Source: CAD feature listing. Evaluate the final solid. Frame: model axes, mm. A direction names the side the tool comes from. Coordinates: 2 decimals unless noted, no trailing zeros. Order: outer loops, then holes, each group sorted by start corner. A loop starts at its lowest first (then second) coordinate and runs counter-clockwise, first axis right, second up. Notation, with made-up numbers: (-37.75, 36.5) -> (-28.75, 36.5) arc R27 ccw to (-28.75, 75.5) -> close; hole circle Ø8 at (-12.75, -26). An arc over 180 degrees is marked (long way). Put each result on its own line as item: value.
from build123d import *

# Parameters (mm, degrees)
SKETCH_1_W                   = 38
SKETCH_1_H                   = 6.45
EXTRUDE_1_DEPTH              = 35
SKETCH_2_W                   = 10
SKETCH_2_H                   = 35
EXTRUDE_2_DEPTH              = 15
HOLE_WIZARD_M4_1_D           = 4.5
HOLE_WIZARD_M4_1_CBORE_D     = 8
HOLE_WIZARD_M4_1_CBORE_DEPTH = 4
PATTERN_LINEAR_1_COUNT       = 2
PATTERN_LINEAR_1_PITCH       = 11
SKETCH_5_R                   = 2
CUT_EXTRUDE_1_DEPTH          = 54.795910625
SKETCH_6_R                   = 2
CUT_EXTRUDE_2_DEPTH          = 56.938381278
PATTERN_LINEAR_2_COUNT       = 2
PATTERN_LINEAR_2_PITCH       = 28
PATTERN_LINEAR_2_COUNT_DIR2  = 2
PATTERN_LINEAR_2_PITCH_DIR2  = 25
CHAMFER_1_SIZE               = 0.5


with BuildPart() as part:
    # 草图1 → 凸台-拉伸1 (new body)
    with BuildSketch(Plane.XY):
        with Locations((19, 3.225)):
            Rectangle(SKETCH_1_W, SKETCH_1_H)
    extrude(amount=EXTRUDE_1_DEPTH)

    # 草图2 → 凸台-拉伸2 (add)
    with BuildSketch(Plane(origin=(0, 6.45, 0), x_dir=(1, 0, 0), z_dir=(0, 1, 0))):
        with Locations((5, -17.5)):
            Rectangle(SKETCH_2_W, SKETCH_2_H)
        with Locations((33, -17.5)):
            Rectangle(SKETCH_2_W, SKETCH_2_H)
    extrude(amount=EXTRUDE_2_DEPTH)

    # Hole Wizard M4 _1 (through all)
    with Locations(Plane(origin=(0, 21.45, 0), x_dir=(-1, 0, 0), z_dir=(0, 1, 0))):
        with Locations((-5, 23)):
            hole_wizard_m4_1 = CounterBoreHole(HOLE_WIZARD_M4_1_D / 2, HOLE_WIZARD_M4_1_CBORE_D / 2, HOLE_WIZARD_M4_1_CBORE_DEPTH)

    # 阵列(线性)1: Hole Wizard M4 _1 ×2
    with Locations(*[(0, 0, -i * PATTERN_LINEAR_1_PITCH) for i in range(1, PATTERN_LINEAR_1_COUNT)]):
        add(hole_wizard_m4_1, mode=Mode.SUBTRACT)

    # 草图5 → 切除-拉伸1 (cut, through all)
    with BuildSketch(Plane(origin=(0, 6.45, 0), x_dir=(1, 0, 0), z_dir=(0, 1, 0))):
        with Locations(Location((19, -27.5, 0), (0, 0, 180))):
            Circle(SKETCH_5_R)
        with Locations(Location((19, -7.5, 0), (0, 0, 180))):
            Circle(SKETCH_5_R)
    extrude(amount=-CUT_EXTRUDE_1_DEPTH, mode=Mode.SUBTRACT)

    # 草图6 → 切除-拉伸2 (cut, through all)
    with BuildSketch(Plane(origin=(0, 21.45, 0), x_dir=(1, 0, 0), z_dir=(0, 1, 0))):
        with Locations(Location((33, -23, 0), (0, 0, 270))):
            Circle(SKETCH_6_R)
        with Locations(Location((33, -12, 0), (0, 0, 270))):
            Circle(SKETCH_6_R)
    extrude(amount=-CUT_EXTRUDE_2_DEPTH, mode=Mode.SUBTRACT)

    # 草图7 → Hole Wizard M4 _1 2 (revolve, cut)
    with BuildSketch(Plane(origin=(5, 21.45, 30), x_dir=(0, 0, 1), z_dir=(1, 0, 0))):
        Polygon((0, 0), (0, 11.091420021), (1.65, 10.1), (1.65, 0), align=None)
    hole_wizard_m4_1_2 = revolve(axis=Axis((5, 27.8, 30), (0, -1, 0)), mode=Mode.SUBTRACT)

    # 阵列(线性)2: Hole Wizard M4 _1 2 2 × 2
    with Locations(*[(i * PATTERN_LINEAR_2_PITCH, 0, -j * PATTERN_LINEAR_2_PITCH_DIR2) for i in range(PATTERN_LINEAR_2_COUNT) for j in range(PATTERN_LINEAR_2_COUNT_DIR2) if (i, j) != (0, 0)]):
        add(hole_wizard_m4_1_2, mode=Mode.SUBTRACT)

    # 倒角1
    chamfer_1_edges = [part.edges().sort_by_distance(p)[0] for p in [
        (5, 21.45, 35),
        (10, 13.95, 35),
        (19, 6.45, 0),
        (19, 6.45, 35),
        (28, 13.95, 35),
        (33, 21.45, 35),
        (19, 0, 0),
        (19, 0, 35),
        (38, 0, 17.5),
        (38, 10.725, 0),
        (38, 10.725, 35),
        (38, 21.45, 17.5),
        (33, 21.45, 0),
        (28, 13.95, 0),
        (10, 13.95, 0),
        (5, 21.45, 0),
        (0, 21.45, 17.5),
        (0, 10.725, 0),
        (0, 10.725, 35),
        (0, 0, 17.5),
    ]]
    chamfer(chamfer_1_edges, length=CHAMFER_1_SIZE)


solid = part.part
1. Pull-direction query (X, two-part tool) for faces 1 (the cylindrical face through (6.21, 8.603, 13.897)), 2 (the flat face through (38, 11, 17)), 3 (the flat face through (0, 11, 18)); classes: pulls with the +X half, pulls with the -X half, needs draft (parallel to the pull), parting line crosses it, or undercut.
Numbers:
face 1: undercut
face 2: pulls with the +X half
face 3: pulls with the -X half
2. Cut plane C-C on z = 7.5. Output: boundary loops of the cut face in (x, y), plus the area to 3 significant figures.
Numbers:
outline: (0, 0.5) -> (0.5, 0) -> (17, 0) -> (17, 6.45) -> (10, 6.45) -> (10, 21.45) -> (0.5, 21.45) -> (0, 20.95) -> close; (21, 0) -> (37.5, 0) -> (38, 0.5) -> (38, 20.95) -> (37.5, 21.45) -> (28, 21.45) -> (28, 6.45) -> (21, 6.45) -> close
area: 519 mm2
3. Cut plane D-D on z = 23. Output: boundary loops of the cut face in (x, y), plus the area to 3 significant figures.
Numbers:
outline: (0, 0.5) -> (0.5, 0) -> (2.75, 0) -> (2.75, 17.45) -> (1, 17.45) -> (1, 21.45) -> (0.5, 21.45) -> (0, 20.95) -> close; (7.25, 0) -> (31, 0) -> (31, 21.45) -> (28, 21.45) -> (28, 6.45) -> (10, 6.45) -> (10, 21.45) -> (9, 21.45) -> (9, 17.45) -> (7.25, 17.45) -> close; (35, 0) -> (37.5, 0) -> (38, 0.5) -> (38, 20.95) -> (37.5, 21.45) -> (35, 21.45) -> close
area: 348 mm2
4. Ray query, line 1 along Z through (x, y) = (5, 11.75); line 2 along X through (y, z) = (16, 30); line 3 along X through (y, z) = (17, 3). Return the intervals inside material, ascending.
Numbers:
line 1: z = 0 to 3.35, 6.65 to 9.75, 14.25 to 20.75, 25.25 to 28.35, 31.65 to 35
line 2: x = 0 to 3.35, 6.65 to 10, 28 to 31.35, 34.65 to 38
line 3: x = 0 to 10, 28 to 38
5. Set-up query: faces 4 (the cylindrical face through (5.521, 19.478, 26.966)), 5 (the flat face through (19, 6.45, 17)), 6 (the flat face through (5, 21.45, 17)). Return all of +Z, -Z, +X, -X, +Y, -Y with unobstructed straight access to the full face (end or side cutting, diameter ignored); none if empty.
Numbers:
face 4: +Y
face 5: +Z, -Z, +Y
face 6: +Z, -Z, +X, -X, +Y
6. First-contact query: pin 1 (3 mm diameter, centred on x = 33, z = 23, fed in from -Y); pin 2 (5 mm diameter, centred on x = 19, z = 27.5, fed in from +Y); pin 3 (7 mm diameter, centred on x = 5, z = 12, fed in from +Y). Flat tips, straight axial feed; report the tip coordinate or a pass-through.
Numbers:
pin 1: passes through
pin 2: stops at y = 6.45
pin 3: stops at y = 17.45
7. Cut plane A-A on y = 15.75. Count the separate pieces of the cut face and the enclosed holes in it, plus the area to 3 significant figures.
Numbers:
separate pieces: 2
enclosed holes: 8
area: 608 mm2
8. Cut plane B-B on x = 19. Output: boundary loops of the cut face in (y, z), plus the area to 3 significant figures.
Numbers:
outline: (0, 0.5) -> (0.5, 0) -> (5.95, 0) -> (6.45, 0.5) -> (6.45, 5.5) -> (0, 5.5) -> close; (0, 9.5) -> (6.45, 9.5) -> (6.45, 25.5) -> (0, 25.5) -> close; (0, 29.5) -> (6.45, 29.5) -> (6.45, 34.5) -> (5.95, 35) -> (0.5, 35) -> (0, 34.5) -> close
area: 174 mm2
